from build123d import *

# Parameters (mm, degrees)
SKETCH_2_R               = 3.9
SKETCH_2_R_2             = 4.1
SKETCH_2_R_3             = 1
SKETCH_2_R_4             = 1.25
EXTRUDE_1_DEPTH          = 3.5
SKETCH_2_4_R             = 4.1
SKETCH_2_4_R_2           = 2.8
EXTRUDE_2_DEPTH          = 1
CUT_EXTRUDE_1_DEPTH      = 41.636067723
CUT_EXTRUDE_1_DEPTH_BACK = 41.636067723
SKETCH_3_W               = 54.4
SKETCH_3_H               = 22
FILLET_1_R               = 10
CUT_EXTRUDE_2_DEPTH      = 36.158071619
CUT_EXTRUDE_2_DEPTH_BACK = 7
SKETCH_4_R               = 1
SKETCH_4_4_R             = 1.5
EXTRUDE_3_DEPTH          = 1.6
SKETCH_5_R               = 1
SKETCH_5_R_2             = 3.9
EXTRUDE_4_DEPTH          = 13
SKETCH_6_R               = 1
SKETCH_6_R_2             = 3.9
CUT_EXTRUDE_3_DEPTH      = 10
CUT_EXTRUDE_4_DEPTH      = 37.51301138
CUT_EXTRUDE_4_DEPTH_BACK = 37.51301138
SKETCH_2_5_R             = 4.1
SKETCH_2_5_R_2           = 2.8
EXTRUDE_5_DEPTH          = 13
SKETCH_8_R               = 4.1
EXTRUDE_6_DEPTH          = 12
EXTRUDE_START            = 9.5
EXTRUDE_7_DEPTH          = 2.5
SKETCH_2_6_R             = 4.1
SKETCH_2_6_R_2           = 2.8
CUT_EXTRUDE_10_DEPTH     = 2.5


# Read off the part's stored shape, not the designer's step: 凸台-拉伸7
with BuildPart() as part:
    # 草图2 → 凸台-拉伸1 (new body)
    with BuildSketch(Plane.XY):
        with BuildLine():
            Line((15.2, -20), (-15.2, -20))
            ThreePointArc((-15.2, -20), (-35.2, 0), (-15.2, 20))
            Line((-15.2, 20), (15.2, 20))
            ThreePointArc((15.2, 20), (35.2, 0), (15.2, -20))
        make_face()
        Circle(SKETCH_2_R, mode=Mode.SUBTRACT)
        with Locations((-15.2, 0)):
            Circle(SKETCH_2_R_2, mode=Mode.SUBTRACT)
        with Locations((15.2, 0)):
            Circle(SKETCH_2_R_2, mode=Mode.SUBTRACT)
        with Locations((-6.2, 0)):
            Circle(SKETCH_2_R_3, mode=Mode.SUBTRACT)
        with Locations((6.2, 0)):
            Circle(SKETCH_2_R_3, mode=Mode.SUBTRACT)
        with Locations((-15.2, 8)):
            Circle(SKETCH_2_R_4, mode=Mode.SUBTRACT)
        with Locations((-23.2, 0)):
            Circle(SKETCH_2_R_4, mode=Mode.SUBTRACT)
        with Locations((23.2, 0)):
            Circle(SKETCH_2_R_4, mode=Mode.SUBTRACT)
        with Locations((15.2, 8)):
            Circle(SKETCH_2_R_4, mode=Mode.SUBTRACT)
    extrude(amount=EXTRUDE_1_DEPTH)

    # 草图2<4> → 凸台-拉伸2 (add)
    # profile 1 of 2: a face of its own
    with BuildSketch(Plane.XY):
        with Locations((-15.2, 0)):
            Circle(SKETCH_2_4_R)
        with Locations((-15.2, 0)):
            Circle(SKETCH_2_4_R_2, mode=Mode.SUBTRACT)
    # profile 2 of 2: a face of its own
    with BuildSketch(Plane.XY):
        with Locations((15.2, 0)):
            Circle(SKETCH_2_4_R)
        with Locations((15.2, 0)):
            Circle(SKETCH_2_4_R_2, mode=Mode.SUBTRACT)
    extrude(amount=EXTRUDE_2_DEPTH)

    # 草图3 → 切除-拉伸1 (cut, two sides: drawn at the far end of the back side and taken through both)
    with BuildSketch(Plane.XY.offset(3.5).offset(-CUT_EXTRUDE_1_DEPTH_BACK)):
        with BuildLine():
            Line((15.2, -20), (-15.2, -20))
            ThreePointArc((-15.2, -20), (-35.2, 0), (-15.2, 20))
            Line((-15.2, 20), (15.2, 20))
            ThreePointArc((15.2, 20), (35.2, 0), (15.2, -20))
        make_face()
        with Locations((0, 1)):
            Rectangle(SKETCH_3_W, SKETCH_3_H, mode=Mode.SUBTRACT)
    extrude(amount=CUT_EXTRUDE_1_DEPTH + CUT_EXTRUDE_1_DEPTH_BACK, mode=Mode.SUBTRACT)

    # 圆角1
    fillet_1_edges = [part.edges().sort_by_distance(p)[0] for p in [
        (27.2, 12, 1.75),
        (-27.2, 12, 1.75),
    ]]
    fillet(fillet_1_edges, radius=FILLET_1_R)

    # 草图4 → 切除-拉伸2 (cut, two sides: drawn at the far end of the back side and taken through both)
    with BuildSketch(Plane.XZ.offset(10).offset(-CUT_EXTRUDE_2_DEPTH_BACK)):
        with Locations(Location((-24, 1.75, 0), (0, 0, 90))):
            Circle(SKETCH_4_R)
        with Locations(Location((24, 1.75, 0), (0, 0, 90))):
            Circle(SKETCH_4_R)
    extrude(amount=CUT_EXTRUDE_2_DEPTH + CUT_EXTRUDE_2_DEPTH_BACK, mode=Mode.SUBTRACT)

    # 草图4<4> → 凸台-拉伸3 (add)
    with BuildSketch(Plane.XZ.offset(10)):
        with Locations(Location((-16, 1.75, 0), (0, 0, 270))):
            Circle(SKETCH_4_4_R)
        with Locations(Location((16, 1.75, 0), (0, 0, 270))):
            Circle(SKETCH_4_4_R)
    extrude(amount=EXTRUDE_3_DEPTH)

    # 草图5 → 凸台-拉伸4 (add)
    with BuildSketch(Plane(origin=(0, 0, 0), x_dir=(-1, 0, 0), z_dir=(0, 0, -1))):
        with BuildLine():
            Line((6.32455532, 9), (-6.32455532, 9))
            ThreePointArc((-6.32455532, 9), (-11, 0), (-6.32455532, -9))
            Line((-6.32455532, -9), (6.32455532, -9))
            ThreePointArc((6.32455532, -9), (9.761406367, -5.070990607), (11, 0))
            ThreePointArc((11, 0), (9.761406367, 5.070990607), (6.32455532, 9))
        make_face()
        with Locations((-6.2, 0)):
            Circle(SKETCH_5_R, mode=Mode.SUBTRACT)
        Circle(SKETCH_5_R_2, mode=Mode.SUBTRACT)
        with Locations((6.2, 0)):
            Circle(SKETCH_5_R, mode=Mode.SUBTRACT)
    extrude(amount=-EXTRUDE_4_DEPTH)

    # 草图6 → 切除-拉伸3 (cut)
    with BuildSketch(Plane(origin=(0, 0, 0), x_dir=(-1, 0, 0), z_dir=(0, 0, -1))):
        with BuildLine():
            Line((6.65, 7.8), (-6.65, 7.8))
            ThreePointArc((-6.65, 7.8), (-10.25, 0), (-6.65, -7.8))
            Line((-6.65, -7.8), (6.65, -7.8))
            ThreePointArc((6.65, -7.8), (9.306583691, -4.295346319), (10.25, 0))
            ThreePointArc((10.25, 0), (9.306583691, 4.295346319), (6.65, 7.8))
        make_face()
        with Locations((-6.2, 0)):
            Circle(SKETCH_6_R, mode=Mode.SUBTRACT)
        Circle(SKETCH_6_R_2, mode=Mode.SUBTRACT)
        with Locations((6.2, 0)):
            Circle(SKETCH_6_R, mode=Mode.SUBTRACT)
    extrude(amount=-CUT_EXTRUDE_3_DEPTH, mode=Mode.SUBTRACT)

    # 草图7 → 切除-拉伸4 (cut, two sides: drawn at the far end of the back side and taken through both)
    with BuildSketch(Plane(origin=(0, 9, 0), x_dir=(1, 0, 0), z_dir=(0, 1, 0)).offset(-CUT_EXTRUDE_4_DEPTH_BACK)):
        with BuildLine():
            Line((-3, -4.5), (3, -4.5))
            ThreePointArc((3, -4.5), (5, -6.5), (3, -8.5))
            Line((3, -8.5), (-3, -8.5))
            ThreePointArc((-3, -8.5), (-5, -6.5), (-3, -4.5))
        make_face()
    extrude(amount=CUT_EXTRUDE_4_DEPTH + CUT_EXTRUDE_4_DEPTH_BACK, mode=Mode.SUBTRACT)

    # 草图2<5> → 凸台-拉伸5 (add)
    # profile 1 of 2: a face of its own
    with BuildSketch(Plane.XY):
        with Locations(Location((-15.2, 0, 0), (0, 0, 180))):
            Circle(SKETCH_2_5_R)
        with Locations((-15.2, 0)):
            Circle(SKETCH_2_5_R_2, mode=Mode.SUBTRACT)
    # profile 2 of 2: a face of its own
    with BuildSketch(Plane.XY):
        with Locations(Location((15.2, 0, 0), (0, 0, 180))):
            Circle(SKETCH_2_5_R)
        with Locations((15.2, 0)):
            Circle(SKETCH_2_5_R_2, mode=Mode.SUBTRACT)
    extrude(amount=EXTRUDE_5_DEPTH)

    # 草图8 → 凸台-拉伸6 (add)
    # profile 1 of 2: a face of its own
    with BuildSketch(Plane.XY.offset(3.5)):
        with BuildLine():
            ThreePointArc((-10.774259868, -2.217053064), (-11, 0), (-10.774259868, 2.217053064))
            ThreePointArc((-10.774259868, 2.217053064), (-20.15, 0), (-10.774259868, -2.217053064))
        make_face()
        with Locations((-15.2, 0)):
            Circle(SKETCH_8_R, mode=Mode.SUBTRACT)
    # profile 2 of 2: a face of its own
    with BuildSketch(Plane.XY.offset(3.5)):
        with BuildLine():
            ThreePointArc((10.774259868, -2.217053064), (16.339097526, -4.817152356), (20.15, 0))
            ThreePointArc((20.15, 0), (16.339097526, 4.817152356), (10.774259868, 2.217053064))
            ThreePointArc((10.774259868, 2.217053064), (11, 0), (10.774259868, -2.217053064))
        make_face()
        with Locations((15.2, 0)):
            Circle(SKETCH_8_R, mode=Mode.SUBTRACT)
    extrude(amount=EXTRUDE_6_DEPTH)

    # 凸台-拉伸7 outline → 凸台-拉伸7 (add)
    with BuildSketch(Plane.XY.offset(3.5).offset(EXTRUDE_START)):
        with BuildLine():
            ThreePointArc((-10.774259868, -2.217053064), (-10.25, 0), (-10.774259868, 2.217053064))
            ThreePointArc((-10.774259868, 2.217053064), (-11, 0), (-10.774259868, -2.217053064))
        make_face()
        with BuildLine():
            ThreePointArc((10.774259868, -2.217053064), (11, 0), (10.774259868, 2.217053064))
            ThreePointArc((10.774259868, 2.217053064), (10.25, 0), (10.774259868, -2.217053064))
        make_face()
    extrude(amount=EXTRUDE_7_DEPTH)

    # 草图2<6> → 切除-拉伸10 (cut)
    # profile 1 of 2: a face of its own
    with BuildSketch(Plane.XY):
        with Locations((-15.2, 0)):
            Circle(SKETCH_2_6_R)
        with Locations((-15.2, 0)):
            Circle(SKETCH_2_6_R_2, mode=Mode.SUBTRACT)
    # profile 2 of 2: a face of its own
    with BuildSketch(Plane.XY):
        with Locations((15.2, 0)):
            Circle(SKETCH_2_6_R)
        with Locations((15.2, 0)):
            Circle(SKETCH_2_6_R_2, mode=Mode.SUBTRACT)
    extrude(amount=CUT_EXTRUDE_10_DEPTH, mode=Mode.SUBTRACT)


solid = part.part
Read the model definition and answer for the solid it produces. Units are mm, in the model's axes. A direction names the side the tool comes from. Round coordinates to 2 decimals unless told otherwise and drop trailing zeros. Order: outer loops, then holes, each group sorted by start corner. A loop starts at its lowest first (then second) coordinate and runs counter-clockwise, first axis right, second up.
1) Flat-ended cylindrical pins translate along their axes: pin 1 (4 mm diameter, centred on x = -14, y = 1.5, fed in from -Z); pin 2 (1 mm diameter, centred on x = 10.5, y = -9, fed in from +Z); pin 3 (10.5 mm diameter, centred on x = -15.2, y = 0, fed in from +Z); pin 4 (6 mm diameter, centred on x = 0, y = 0, fed in from +Z). Find the tip coordinate at first contact, or state that the pin passes through.
2) The part is cut by section B-B on x = -15.5. Write down the section's boundary in (y, z), plus the area to 3 significant figures.
3) The part is cut by section C-C on y = -6.25. Write down the section's boundary in (x, z), plus the area to 3 significant figures.
4) The part is cut by section D-D on z = 8. Write down the section's boundary in (x, y), plus the area to 3 significant figures.
5) For faces 4 (the face through (17.01, -10.79, 2.86)), 5 (the face through (0, 9, 9)), 6 (the face through (0, -8, 8.5)), 7 (the face through (0, 7.8, 4)), determine the directions among +Z, -Z, +X, -X, +Y, -Y from which every point of the face is accessible in a straight line to the end or side of a thin tool.
6) Straight lines are drawn through the part: L1, parallel to Y at x = 15.2, z = 1.05; L2, parallel to X at y = 0, z = 14.2; L3, parallel to Y at x = -23.2, z = 0.8. For each, find the intervals that lie inside material, in ascending order.
7) The mould has two halves that part along X. Classify faces 1 (the face through (24.976, -6.451, 1.533)), 2 (the face through (-27.2, -4, 2)), 3 (the face through (-17, 4, 15.5)): released by +X, released by -X, zero draft, split by the parting line, or undercut.
8) The part is cut by section A-A on z = 1.75. Give the number of separate pieces and of enclosed holes in the cut face, plus the area to 3 significant figures.
Resolved:
1. pin 1: stops at z = 2.5
1. pin 2: stops at z = 3.5
1. pin 3: stops at z = 15.5
1. pin 4: passes through
2. outline: (-11.6, 0.34) - (-10, 0.34) - (-10, 0) - (-4.09, 0) - (-4.09, 2.5) - (-2.78, 2.5) - (-2.78, 13) - (-4.09, 13) - (-4.09, 15.5) - (-4.94, 15.5) - (-4.94, 3.5) - (-10, 3.5) - (-10, 3.16) - (-11.6, 3.16) - close; (2.78, 2.5) - (4.09, 2.5) - (4.09, 0) - (6.79, 0) - (6.79, 3.5) - (4.94, 3.5) - (4.94, 15.5) - (4.09, 15.5) - (4.09, 13) - (2.78, 13) - close; (9.21, 0) - (12, 0) - (12, 3.5) - (9.21, 3.5) - close
2. area: 92.3 mm2
3. outline: (-27.2, 0) - (-8.12, 0) - (-8.12, 10) - (8.12, 10) - (8.12, 0) - (27.2, 0) - (27.2, 3.5) - (9.05, 3.5) - (9.05, 13) - (-9.05, 13) - (-9.05, 3.5) - (-27.2, 3.5) - close; hole circle Ø2 at (-24, 1.75); hole circle Ø2 at (24, 1.75)
3. area: 194 mm2
4. outline: (-10.77, -2.22) arc R11 ccw to (-6.32, -9) - (-4.32, -9) - (-4.32, -7.8) - (-6.65, -7.8) arc R10.25 cw to (-6.65, 7.8) - (-4.32, 7.8) - (-4.32, 9) - (-6.32, 9) arc R11 ccw to (-10.77, 2.22) arc R4.95 ccw (long way) to start; (4.32, -9) - (6.32, -9) arc R11 ccw to (10.77, -2.22) arc R4.95 ccw (long way) to (10.77, 2.22) arc R11 ccw to (6.32, 9) - (4.32, 9) - (4.32, 7.8) - (6.65, 7.8) arc R10.25 cw to (6.65, -7.8) - (4.32, -7.8) - close; hole circle Ø5.6 at (-15.2, 0); hole circle Ø5.6 at (15.2, 0)
4. area: 140 mm2
5. face 4: -Y
5. face 5: +Z, +X, -X, +Y
5. face 6: +Y, -Y
5. face 7: -Z
6. L1: y = -11.6 to -4.1, 4.1 to 6.75, 9.25 to 12
6. L2: x = -20.15 to -19.3, -11.1 to -10.25, 10.25 to 11.1, 19.3 to 20.15
6. L3: y = -10 to -1.25, 1.25 to 10
7. face 1: undercut
7. face 2: released by -X
7. face 3: zero draft
8. separate pieces: 1
8. enclosed holes: 7
8. area: 725 mm2
